Check sheet for the modelled part. Datum: model origin and axes. Units: mm. A direction names the side the tool comes from. Give positions to 0.01 mm unless a question says otherwise; leave off trailing zeros. Order: outer loops, then holes, each group sorted by start corner. A loop starts at its lowest first (then second) coordinate and runs counter-clockwise, first axis right, second up.
Item 1: Material ranges on line 1 along Y through (x, z) = (0, 8); line 2 along Y through (x, z) = (0, 1.2); line 3 along Z through (x, y) = (-5.5, -4), recorded low to high.
Item 2: Release check for a two-part mould opening along X. For faces 1 (the cylindrical face through (0.715, -1.375, 1.014)), 2 (the flat face through (-8, -7, 9)), 3 (the cylindrical face through (-1.5, 11.4, 4.4)) record: released by +X, released by -X, zero draft, split by the parting line, or undercut.
Item 3: Access from +Z, -Z, +X, -X, +Y, -Y to the whole of each face (thin tool, end or side, straight path). Record for faces 4 (the flat face through (0, -2, 0)), 5 (the cylindrical face through (-2.222, -10.006, 5.451)).
Item 4: Sectioned sample at D-D on x = 7. Record the boundary of the cut face in (y, z).
Item 5: Gauge pin test, flat ends, axial feed: P1, Ø5, axis at y = 6, z = 2.5, coming from the +X side; P2, Ø6, axis at x = 1, y = 1.5, coming from the +Z side. Record the tip position at first contact, or that the pin passes through.
Item 6: Sectioned sample at A-A on x = 0. Record the boundary of the cut face in (y, z).
Item 7: Sectioned sample at C-C on z = 1. Record the boundary of the cut face in (x, y), and give its area (3 significant figures).
from build123d import *

# Parameters (mm, degrees)
F0_R     = 11.5
F1_DEPTH = 2
F2_R     = 11.5
F2_R_2   = 10.25
F3_DEPTH = 7
F2_R_3   = 1.55
F4_DEPTH = 25


with BuildPart() as f1:
    # F0 (on Top) → F1 (new body)
    with BuildSketch(Plane.XY):
        Circle(F0_R)
    extrude(amount=F1_DEPTH)

    # F2 (on face) → F3 (join)
    with BuildSketch(Plane.XY.offset(2)):
        Circle(F2_R)
        Circle(F2_R_2, mode=Mode.SUBTRACT)
    extrude(amount=F3_DEPTH)

    # F2 (on face) → F4 (cut)
    with BuildSketch(Plane.XY.offset(2)):
        Circle(F2_R_3)
    extrude(amount=-F4_DEPTH, mode=Mode.SUBTRACT)


solid = f1.part
Report:
1. line 1: y = -11.5 to -10.25, 10.25 to 11.5
1. line 2: y = -11.5 to -1.55, 1.55 to 11.5
1. line 3: z = 0 to 2
2. face 1: undercut
2. face 2: zero draft
2. face 3: split by the parting line
3. face 4: -Z, +X, -X, +Y, -Y
3. face 5: +Z
4. outline: (-9.12, 0) - (9.12, 0) - (9.12, 9) - (7.49, 9) - (7.49, 2) - (-7.49, 2) - (-7.49, 9) - (-9.12, 9) - close
5. P1: stops at x = 10.95
5. P2: stops at z = 2
6. outline: (-11.5, 0) - (-1.55, 0) - (-1.55, 2) - (-10.25, 2) - (-10.25, 9) - (-11.5, 9) - close; (1.55, 0) - (11.5, 0) - (11.5, 9) - (10.25, 9) - (10.25, 2) - (1.55, 2) - close
7. outline: circle Ø23 at (0, 0); hole circle Ø3.1 at (0, 0)
7. area: 408 mm2
